Geometry: final body of the model. Coordinates: model frame, mm. A direction names the side the tool comes from. Round coordinates to 2 decimals unless told otherwise and drop trailing zeros. Loops run counter-clockwise (first coordinate to the right, second up) from the corner with the lowest first, then second, coordinate; pieces in that order, holes last. Notation, with made-up numbers: M 68.25,-8 L 76.25,-8 A22 cw 76.25,20 Z; hole C 57.25,34.25 d7. An arc over 180 degrees is marked long. Write each question's results on one line, items separated by ' | '.
```python
from build123d import *

# Parameters (mm, degrees)
ESQUISSE2_W        = 6
ESQUISSE2_H        = 24
ESQUISSE2_R        = 1.5
BOSS_EXTRU_2_DEPTH = 2
CONG_2_R           = 2
ESQUISSE3_R        = 3
ESQUISSE3_R_2      = 1.5
BOSS_EXTRU_3_DEPTH = 2


with BuildPart() as part:
    # Esquisse2 → Boss.-Extru.2 (new body)
    with BuildSketch(Plane.XY):
        Rectangle(ESQUISSE2_W, ESQUISSE2_H)
        with Locations((0, 9)):
            Circle(ESQUISSE2_R, mode=Mode.SUBTRACT)
        with Locations((0, -9)):
            Circle(ESQUISSE2_R, mode=Mode.SUBTRACT)
    extrude(amount=BOSS_EXTRU_2_DEPTH)

    # Congé2
    cong_2_edges = [part.edges().sort_by_distance(p)[0] for p in [
        (3, -12, 1),
        (-3, -12, 1),
        (-3, 12, 1),
        (3, 12, 1),
    ]]
    fillet(cong_2_edges, radius=CONG_2_R)

    # Esquisse3 → Boss.-Extru.3 (add)
    # profile 1 of 3: a face of its own
    with BuildSketch(Plane(origin=(0, 0, 0), x_dir=(-1, 0, 0), z_dir=(0, 0, -1))):
        with Locations((0, -9)):
            Circle(ESQUISSE3_R)
        with Locations((0, -9)):
            Circle(ESQUISSE3_R_2, mode=Mode.SUBTRACT)
    # profile 2 of 3: a face of its own
    with BuildSketch(Plane(origin=(0, 0, 0), x_dir=(-1, 0, 0), z_dir=(0, 0, -1))):
        with BuildLine():
            ThreePointArc((3, -9), (2.121320344, -11.121320344), (0, -12))
            Line((0, -12), (1, -12))
            ThreePointArc((1, -12), (2.414213562, -11.414213562), (3, -10))
            Line((3, -10), (3, -9))
        make_face()
    # profile 3 of 3: a face of its own
    with BuildSketch(Plane(origin=(0, 0, 0), x_dir=(-1, 0, 0), z_dir=(0, 0, -1))):
        with BuildLine():
            ThreePointArc((-3, -10), (-2.414213562, -11.414213562), (-1, -12))
            Line((-1, -12), (0, -12))
            ThreePointArc((0, -12), (-2.121320344, -11.121320344), (-3, -9))
            Line((-3, -9), (-3, -10))
        make_face()
    extrude(amount=BOSS_EXTRU_3_DEPTH)


solid = part.part
```
1. Section A-A (y = 9). Output: boundary loops of the cut face in (x, z), then the cut area to 3 significant figures.
Answer key:
outline: M -3,0 L -1.5,0 L -1.5,2 L -3,2 Z; M 1.5,0 L 3,0 L 3,2 L 1.5,2 Z | area: 6.00 mm²
2. Draft query along X for faces 3 (the face through (-3, 0, 1)), 4 (the face through (-0.325, 7.536, 0.986)), 5 (the face through (2.43, -11.4, 0.03)). Return one class per face: pulls with the +X half, pulls with the -X half, needs draft (parallel to the pull), parting line crosses it, or undercut.
Answer key:
face 3: pulls with the -X half | face 4: undercut | face 5: pulls with the +X half
3. Section C-C (x = 0). Output: boundary loops of the cut face in (y, z), then the cut area to 3 significant figures.
Answer key:
outline: M -12,-2 L -10.5,-2 L -10.5,2 L -12,2 Z; M -7.5,-2 L -6,-2 L -6,0 L 7.5,0 L 7.5,2 L -7.5,2 Z; M 10.5,0 L 12,0 L 12,2 L 10.5,2 Z | area: 42.0 mm²
4. Access query for faces 1 (the face through (-2.43, 11.4, 1.01)), 2 (the face through (0, -6, -1)). Directions: +Z, -Z, +X, -X, +Y, -Y. A direction counts if a zero-diameter tool reaches every point of the face in a straight line with its end or side. Return the directions, or none.
Answer key:
face 1: +Z, -Z, -X, +Y | face 2: -Z, +Y
5. Section B-B (z = -1.45). Output: boundary loops of the cut face in (x, y), then the cut area to 3 significant figures.
Answer key:
outline: M -3,-10 A2 ccw -1,-12 L 1,-12 A2 ccw 3,-10 L 3,-9 A3 ccw -3,-9 Z; hole C 0,-9 d3 | area: 23.4 mm²
6. Section D-D (z = 1.15). Output: boundary loops of the cut face in (x, y).
Answer key:
outline: M -3,-10 A2 ccw -1,-12 L 1,-12 A2 ccw 3,-10 L 3,10 A2 ccw 1,12 L -1,12 A2 ccw -3,10 Z; hole C 0,-9 d3; hole C 0,9 d3
7. Ray query, probe 1 along Y at (x, z) = (0, 1.35); probe 2 along X at (y, z) = (-9, 1.5); probe 3 along Y at (x, z) = (-1.25, 1.5). Return the intervals inside material, ascending.
Answer key:
probe 1: y = -12 to -10.5, -7.5 to 7.5, 10.5 to 12 | probe 2: x = -3 to -1.5, 1.5 to 3 | probe 3: y = -11.98 to -9.83, -8.17 to 8.17, 9.83 to 11.98
8. Pin query (flat end, axial travel): P1, Ø1.8, axis at x = -1, y = 5.5, coming from the -Z side; P2, Ø1, axis at x = 2, z = -1.5, coming from the -Y side. Return the tip coordinate at first contact, or that it passes through.
Answer key:
P1: stops at z = 0 | P2: stops at y = -11.94
